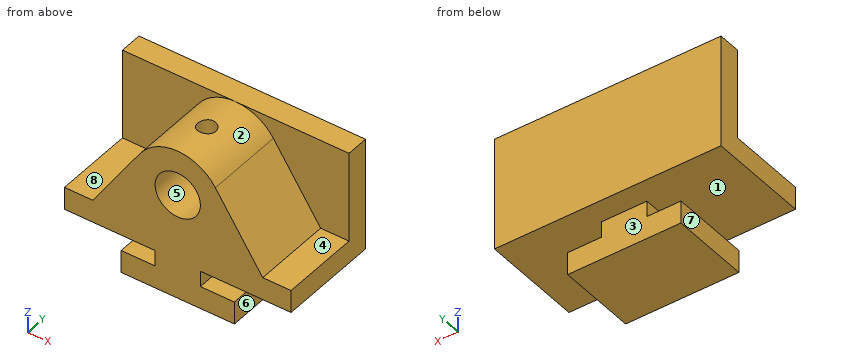
from build123d import *

# Parameters (mm, degrees)
F0_R     = 12.7
F1_DEPTH = 44.45
F2_W     = 12.7
F2_H     = 63.5
F3_DEPTH = 127
F5_R     = 5.08
F6_DEPTH = 25.4


with BuildPart() as f1:
    # F0 (on Front) → F1 (new body)
    with BuildSketch(Plane.XZ):
        with BuildLine():
            Line((-31.75, 0), (0, 0))
            Line((0, 0), (31.75, 0))
            Line((31.75, 0), (31.75, 12.7))
            Line((31.75, 12.7), (12.7, 12.7))
            Line((12.7, 12.7), (12.7, 21.59))
            Line((12.7, 21.59), (63.5, 21.59))
            Line((63.5, 21.59), (63.5, 34.29))
            Line((63.5, 34.29), (47.625, 34.29))
            Line((47.625, 34.29), (21.093426, 73.840173))
            ThreePointArc((21.093426, 73.840173), (0, 85.09), (-21.093426, 73.840173))
            Line((-21.093426, 73.840173), (-47.625, 34.29))
            Line((-47.625, 34.29), (-63.5, 34.29))
            Line((-63.5, 34.29), (-63.5, 21.59))
            Line((-63.5, 21.59), (-12.7, 21.59))
            Line((-12.7, 21.59), (-12.7, 12.7))
            Line((-12.7, 12.7), (-31.75, 12.7))
            Line((-31.75, 12.7), (-31.75, 0))
        make_face()
        with Locations((0, 59.69)):
            Circle(F0_R, mode=Mode.SUBTRACT)
    extrude(amount=F1_DEPTH)

    # F2 (on face) → F3 (join)
    with BuildSketch(Plane.YZ.offset(63.5)):
        with Locations((6.35, 53.34)):
            Rectangle(F2_W, F2_H)
    extrude(amount=-F3_DEPTH)

    # F5 (on offset) → F6 (cut)
    with BuildSketch(Plane.XY.offset(85.09)):
        with Locations((0, -22.225)):
            Circle(F5_R)
    extrude(amount=-F6_DEPTH, mode=Mode.SUBTRACT)


solid = f1.part
Here's how the part is built. I have some questions about the finished solid (model axes, mm). Face numbers are marked on the shaded views. A direction names the side the tool comes from. Give positions to 0.01 mm unless a question says otherwise; leave off trailing zeros. Order: outer loops, then holes, each group sorted by start corner. A loop starts at its lowest first (then second) coordinate and runs counter-clockwise, first axis right, second up. Notation, with made-up numbers: (78.5, -27.5) -> (116.5, -27.5) arc R19 cw to (116.5, 4.5) -> close; hole circle Ø8 at (-24.5, 22). An arc over 180 degrees is marked (long way). One line per item, written item: value. Start each with the question number.
1. Imagine slicing it at D-D, the plane z = 61.5. List the corners of the cut face in (x, y) for me.
2. I need wall thicknesses on probe 1 along Z at (x, y) = (0, -17); probe 2 along Y at (x, z) = (0, 79.75) (3 decimals); probe 3 along Y at (x, z) = (1.5, 59). Which ranges of each line are inside material? Lowest first, please. Write a range as from..to.
3. Imagine slicing it at C-C, the plane z = 77. List the corners of the cut face in (x, y) for me (3 decimals).
4. For the marked faces 4, 5, 6, 7 and 8, which set-ups out of +Z, -Z, +X, -X, +Y, -Y let a thin tool reach every point of the face, with its end or its side?
5. Imagine slicing it at B-B, the plane y = -5. List the corners of the cut face in (x, z) for me (3 decimals).
6. We'd pull the mould along Z, two halves only. Please class the marked faces 1, 2 and 3: released by +Z, released by -Z, zero draft, split by the parting line, or undercut.
7. Will these pins go through, and if not, where does the flat tip stop? pin 1 Ø2 at (x, y) = (39.5, -4.5) entering from -Z; pin 2 Ø9.5 at (x, y) = (-18.5, -30) entering from +Z; pin 3 Ø2.5 at (y, z) = (-15.5, 17) entering from -X.
8. Imagine slicing it at A-A, the plane x = 17. List the corners of the cut face in (y, z) for me.
Values follow:
1. outline: (-63.5, 0) -> (-29.37, 0) -> (-29.37, -44.45) -> (-12.57, -44.45) -> (-12.57, 0) -> (12.57, 0) -> (12.57, -44.45) -> (29.37, -44.45) -> (29.37, 0) -> (63.5, 0) -> (63.5, 12.7) -> (-63.5, 12.7) -> close
2. probe 1: z = 0..46.99, 72.39..85.09
2. probe 2: y = -44.45..-27.305, -17.145..12.7
2. probe 3: y = 0..12.7
3. outline: (-63.5, 0) -> (-18.588, 0) -> (-18.588, -44.45) -> (18.588, -44.45) -> (18.588, 0) -> (63.5, 0) -> (63.5, 12.7) -> (-63.5, 12.7) -> close; hole circle Ø10.16 at (0, -22.225)
4. face 4: +Z, +X, -Y
4. face 5: -Y
4. face 6: -Z, +X, +Y, -Y
4. face 7: -Z, -X, +Y, -Y
4. face 8: +Z, -X, -Y
5. outline: (-63.5, 21.59) -> (-12.7, 21.59) -> (-12.7, 12.7) -> (-31.75, 12.7) -> (-31.75, 0) -> (31.75, 0) -> (31.75, 12.7) -> (12.7, 12.7) -> (12.7, 21.59) -> (63.5, 21.59) -> (63.5, 34.29) -> (47.625, 34.29) -> (21.093, 73.84) arc R25.4 ccw to (-21.093, 73.84) -> (-47.625, 34.29) -> (-63.5, 34.29) -> close; hole circle Ø25.4 at (0, 59.69)
6. face 1: undercut
6. face 2: released by +Z
6. face 3: zero draft
7. pin 1: stops at z = 21.59
7. pin 2: stops at z = 81.05
7. pin 3: stops at x = -12.7
8. outline: (-44.45, 0) -> (0, 0) -> (0, 12.7) -> (-44.45, 12.7) -> close; (-44.45, 21.59) -> (12.7, 21.59) -> (12.7, 85.09) -> (0, 85.09) -> (0, 78.56) -> (-44.45, 78.56) -> close
